```python
from build123d import *

# Parameters (mm, degrees)
SKETCH1_W           = 22.5
SKETCH1_H           = 12.5
BOSS_EXTRUDE1_DEPTH = 22.5
BOSS_EXTRUDE2_START = 17
SKETCH1_3_W         = 4.8
SKETCH1_3_H         = 12.5
SKETCH1_3_W_2       = 4.7
BOSS_EXTRUDE2_DEPTH = 2.5
SKETCH2_R           = 2.5
SKETCH2_R_2         = 6.25
BOSS_EXTRUDE3_DEPTH = 4.25
SKETCH2_3_R         = 2.5
BOSS_EXTRUDE4_DEPTH = 6.75
SKETCH3_W           = 4
SKETCH3_H           = 1.25
BOSS_EXTRUDE5_DEPTH = 10


with BuildPart() as part:
    # Sketch1 → Boss-Extrude1 (new body)
    with BuildSketch(Plane(origin=(0, 0, 0), x_dir=(1, 0, 0), z_dir=(0, 1, 0))):
        with Locations((11.25, 6.25)):
            Rectangle(SKETCH1_W, SKETCH1_H)
    extrude(amount=BOSS_EXTRUDE1_DEPTH)

    # Sketch1_3 → Boss-Extrude2 (add)
    with BuildSketch(Plane(origin=(0, 0, 0), x_dir=(1, 0, 0), z_dir=(0, 1, 0)).offset(BOSS_EXTRUDE2_START)):
        with Locations((-2.4, 6.25)):
            Rectangle(SKETCH1_3_W, SKETCH1_3_H)
        with Locations((24.85, 6.25)):
            Rectangle(SKETCH1_3_W_2, SKETCH1_3_H)
    extrude(amount=BOSS_EXTRUDE2_DEPTH)

    # Sketch2 → Boss-Extrude3 (add)
    with BuildSketch(Plane(origin=(0, 22.5, 0), x_dir=(1, 0, 0), z_dir=(0, 1, 0))):
        with Locations((6.25, 6.25)):
            Circle(SKETCH2_R)
        with Locations((6.25, 6.25)):
            Circle(SKETCH2_R_2)
        with Locations((6.25, 6.25)):
            Circle(SKETCH2_R, mode=Mode.SUBTRACT)
    extrude(amount=BOSS_EXTRUDE3_DEPTH)

    # Sketch2_3 → Boss-Extrude4 (add)
    with BuildSketch(Plane(origin=(0, 22.5, 0), x_dir=(1, 0, 0), z_dir=(0, 1, 0))):
        with Locations((6.25, 6.25)):
            Circle(SKETCH2_3_R)
    extrude(amount=BOSS_EXTRUDE4_DEPTH)

    # Sketch3 → Boss-Extrude5 (add)
    with BuildSketch(Plane.ZY):
        with Locations((-6.25, 4.925)):
            Rectangle(SKETCH3_W, SKETCH3_H)
    extrude(amount=BOSS_EXTRUDE5_DEPTH)


solid = part.part
```
Geometry check sheet. Reference: the model listing, model coordinates, mm. A direction names the side the tool comes from. Round coordinates to 2 decimals unless told otherwise and drop trailing zeros. Loops run counter-clockwise (first coordinate to the right, second up) from the corner with the lowest first, then second, coordinate; pieces in that order, holes last. Notation, with made-up numbers: M 55.5,59.25 L 77.5,59.25 A29 cw 77.5,85.25 Z; hole C 43,89.5 d6. An arc over 180 degrees is marked long. Return JSON: item names as keys, results as strings. Group by question number.
(1) Go/stop test with flat-tipped pins: pin 1 (2.5 mm diameter, centred on y = 21.5, z = -6, fed in from +X); pin 2 (2.5 mm diameter, centred on x = -3, z = -7.5, fed in from +Y); pin 3 (4 mm diameter, centred on y = 9, z = -6.5, fed in from -X). Record where each tip stops, or that it passes through.
(2) Section check A-A, the plane x = 17. Enter the section's corners in (y, z), and give its area (3 significant figures).
(3) Set-up check for faces 1 (the face through (1.29, 24.6, -2.45)), 2 (the face through (0, 21, -6)), 3 (the face through (25, 17, -6)): record each of +Z, -Z, +X, -X, +Y, -Y from which the full face is reachable in a straight line by a thin tool's end or side.
(4) Mould release check, pull along Y, two halves, no side actions. Record for faces 4 (the face through (25, 19.5, -6)), 5 (the face through (22.5, 8, -6)), 6 (the face through (-5, 5.55, -6)), 7 (the face through (-2, 17, -6)): pulls with the +Y half, pulls with the -Y half, needs draft (parallel to the pull), parting line crosses it, or undercut.
(5) Section check D-D, the plane y = 25.75. Enter the section's corners in (x, z), and give its area (3 significant figures).
(6) Section check C-C, the plane z = -7. Enter the section's corners in (x, y), and give its area (3 significant figures).
(7) Scan lines: line 1 along X through (y, z) = (7.75, -3.75); line 2 along Y through (x, z) = (2, -7). Record each from-to range of solid material in increasing order. Write a range as [from, to].
(8) Section check B-B, the plane y = 18. Enter the section's corners in (x, z).
Data:
{
 "1": {"pin 1": "x = 22.5", "pin 2": "y = 19.5", "pin 3": "x = 0"},
 "2": {"outline": "M 0,-12.5 L 22.5,-12.5 L 22.5,0 L 0,0 Z", "area": "281 mm²"},
 "3": {"face 1": "+Y", "face 2": "+Z, -Z, -X, +Y", "face 3": "+Z, -Z, +X, -Y"},
 "4": {"face 4": "pulls with the +Y half", "face 5": "needs draft", "face 6": "undercut", "face 7": "undercut"},
 "5": {"outline": "C 6.25,-6.25 d12.5", "area": "123 mm²"},
 "6": {"outline": "M -10,4.3 L 0,4.3 L 0,0 L 22.5,0 L 22.5,17 L 27.2,17 L 27.2,19.5 L 22.5,19.5 L 22.5,22.5 L 12.45,22.5 L 12.45,26.75 L 8.63,26.75 L 8.63,29.25 L 3.87,29.25 L 3.87,26.75 L 0.05,26.75 L 0.05,22.5 L 0,22.5 L 0,19.5 L -4.8,19.5 L -4.8,17 L 0,17 L 0,5.55 L -10,5.55 Z", "area": "607 mm²"},
 "7": {"line 1": "[0, 22.5]", "line 2": "[0, 26.75]"},
 "8": {"outline": "M -4.8,-12.5 L 27.2,-12.5 L 27.2,0 L -4.8,0 Z"}
}
